Geometry check sheet. Reference: the model listing, model coordinates, mm. Coordinates: 2 decimals unless noted, no trailing zeros. Loops run counter-clockwise (first coordinate to the right, second up) from the corner with the lowest first, then second, coordinate; pieces in that order, holes last.
Autodesk Inventor part; units mm, degrees
ref_plane "YZ Plane" through (0, 0, 0) normal (1, 0, 0) x (0, 1, 0)
ref_plane "XZ Plane" through (0, 0, 0) normal (0, 1, 0) x (-1, 0, 0)
ref_plane "XY Plane" through (0, 0, 0) normal (0, 0, 1) x (1, 0, 0)
sketch "Sketch1" plane through (0, 0, 0) normal (0, 1, 0) x (-1, 0, 0)
  line L0 (-40, 417.5) -> (40, 417.5)
  line L1 (40, 417.5) -> (40, -417.5)
  line L2 (40, -417.5) -> (-40, -417.5)
  line L3 (-40, -417.5) -> (-40, 417.5)
  line L4 (-40, 417.5) -> (40, -417.5) construction
  line L5 (40, 417.5) -> (-40, -417.5) construction
  point P0 (0, 0)
  dimension "d0" = 80
  dimension "d1" = 835
extrude "Extrusion1" add sketch "Sketch1" along normal blind 12
fillet "Fillet1" radius 2 1 edges at (40, 6, 417.5)
fillet "Fillet2" radius 2 3 edges at (39.4142, 12, 416.9142) (-1, 12, 417.5) (40, 12, -1)
fillet "Fillet3" radius 2 3 edges at (39.4142, 0, 416.9142) (-1, 0, 417.5) (40, 0, -1)
fillet "Fillet4" radius 2 5 edges at (-40, 6, 417.5) (-40, 0.5858, 416.9142) (-40, 0, -1) (-40, 12, -1) (-40, 11.4142, 416.9142)
fillet "Fillet5" radius 2 8 edges at (-39.4142, 11.4142, -417.5) (0, 12, -417.5) (39.4142, 11.4142, -417.5) (40, 6, -417.5) (39.4142, 0.5858, -417.5) (0, 0, -417.5) (-39.4142, 0.5858, -417.5) (-40, 6, -417.5)
sketch "Sketch2" plane through (-40, 2, -415.5) normal (-1, 0, 0) x (0, 0, 1)
  circle A0 centre (18, 4) radius 4
  line L0 (-2, 8) -> (-2, 0)
  line L1 (0, -2) -> (831, -2)
  circle A1 centre (813, 4) radius 4
  line L2 (833, 0) -> (833, 8)
  line L3 (831, 10) -> (0, 10)
  point P0 (415.5, -2)
  dimension "d9" = 8
  dimension "d10" = 20
  dimension "d11" = 6
  dimension "d12" = 8
  dimension "d13" = 20
  dimension "d21" = 6
hole "Hole1" at (-40, 6, -397.5) at (-40, 6, 397.5) direction (1, 0, 0) diameter 8 end through all
equation "\"d12\" = d9"
equation "\"d13\" = d10"
equation "\"d21\" = d11"
properties part number "CeramicModelv2"
1) Section check A-A on y = 6. Record the cut outline in (x, z).
Data:
outline: (-40, -415.5) arc R2 ccw to (-38, -417.5) - (38, -417.5) arc R2 ccw to (40, -415.5) - (40, -401.5) - (-40, -401.5) - close; (-40, -393.5) - (40, -393.5) - (40, 393.5) - (-40, 393.5) - close; (-40, 401.5) - (40, 401.5) - (40, 415.5) arc R2 ccw to (38, 417.5) - (-38, 417.5) arc R2 ccw to (-40, 415.5) - close
2) Depth check by flat-ended pin: pin 1 (5 mm diameter, centred on y = 6, z = 397.5, fed in from -X). Enter the tip coordinate at first touch or a pass-through.
Data:
pin 1: passes through
3) Material ranges on probe 1 along Z at (x, y) = (20.5, 6); probe 2 along Y at (x, z) = (-14, -397.5); probe 3 along Z at (x, y) = (-16.5, 9.25), recorded low to high.
Data:
probe 1: z = -417.5 to -401.5, -393.5 to 393.5, 401.5 to 417.5
probe 2: y = 0 to 2, 10 to 12
probe 3: z = -417.5 to -399.83, -395.17 to 395.17, 399.83 to 417.5
